```python
from build123d import *

# Parameters (mm, degrees)
SKETCH1_W           = 65
SKETCH1_H           = 16
BOSS_EXTRUDE1_DEPTH = 2
SKETCH2_W           = 65
SKETCH2_H           = 16
SKETCH2_W_2         = 61
SKETCH2_H_2         = 12
BOSS_EXTRUDE2_DEPTH = 2
SKETCH4_W           = 65
SKETCH4_H           = 16
SKETCH4_W_2         = 61
SKETCH4_H_2         = 8
BOSS_EXTRUDE3_DEPTH = 2
SKETCH5_R           = 1
CUT_EXTRUDE1_DEPTH  = 1


with BuildPart() as part:
    # Sketch1 → Boss-Extrude1 (new body)
    with BuildSketch(Plane.XY):
        Rectangle(SKETCH1_W, SKETCH1_H)
    extrude(amount=BOSS_EXTRUDE1_DEPTH)

    # Sketch2 → Boss-Extrude2 (add)
    with BuildSketch(Plane.XY.offset(2)):
        Rectangle(SKETCH2_W, SKETCH2_H)
        Rectangle(SKETCH2_W_2, SKETCH2_H_2, mode=Mode.SUBTRACT)
    extrude(amount=BOSS_EXTRUDE2_DEPTH)

    # Sketch4 → Boss-Extrude3 (add)
    with BuildSketch(Plane.XY.offset(4)):
        Rectangle(SKETCH4_W, SKETCH4_H)
        Rectangle(SKETCH4_W_2, SKETCH4_H_2, mode=Mode.SUBTRACT)
    extrude(amount=BOSS_EXTRUDE3_DEPTH)

    # Sketch5 → Cut-Extrude1 (cut)
    with BuildSketch(Plane.XY.offset(2)):
        with Locations((-26.5, 0)):
            Circle(SKETCH5_R)
    extrude(amount=-CUT_EXTRUDE1_DEPTH, mode=Mode.SUBTRACT)


solid = part.part
```
Design review of the part built by this model. Coordinates are the model's own, in mm. A direction names the side the tool comes from. Round coordinates to 2 decimals unless told otherwise and drop trailing zeros. Write each loop counter-clockwise with the first axis right and the second up, starting at its lowest first coordinate (ties: lowest second). Pieces come first, ordered by that corner, then holes. Notation, with made-up numbers: (-35.75, -38.75) -> (1.25, -38.75) arc R14 cw to (1.25, -31.75) -> close; hole circle Ø3 at (-25, 38.5). An arc over 180 degrees is marked (long way). Answer in a Markdown table with one row per item.
Q1. Clearance check with a flat-ended pin moving along its axis: pin 1 Ø1 at (x, y) = (-26.5, 0) entering from +Z. State where the tip first meets the part, or that it passes through.
The answers:
| item | result |
|---|---|
| pin 1 | z = 1 |
Q2. To check wall thickness, follow L1, parallel to Y at x = 12.5, z = 2.8; L2, parallel to Z at x = -20.5, y = -5; L3, parallel to Y at x = -26.5, z = 1.7. State the ranges of each line that lie inside material, in increasing order. Write a range as [from, to].
The answers:
| item | result |
|---|---|
| L1 | [-8, -6], [6, 8] |
| L2 | [0, 2], [4, 6] |
| L3 | [-8, -1], [1, 8] |
Q3. Take a section at A-A, the plane y = -3. State the section outline as (x, z) points, then the cut area to 3 significant figures.
The answers:
| item | result |
|---|---|
| outline | (-32.5, 0) -> (32.5, 0) -> (32.5, 6) -> (30.5, 6) -> (30.5, 2) -> (-30.5, 2) -> (-30.5, 6) -> (-32.5, 6) -> close |
| area | 146 mm² |
Q4. For faces 1 (the face through (0, 5, 4)), 2 (the face through (-27.5, 0, 1.5)), 3 (the face through (-32.5, 0, 3)), list the 3-axis set-ups (+Z, -Z, +X, -X, +Y, -Y) from which the entire face can be reached by the end or side of a thin tool; tool diameter is ignored.
The answers:
| item | result |
|---|---|
| face 1 | none |
| face 2 | +Z |
| face 3 | +Z, -Z, -X, +Y, -Y |
Q5. Take a section at C-C, the plane x = -26.5. State the section outline as (y, z) points.
The answers:
| item | result |
|---|---|
| outline | (-8, 0) -> (8, 0) -> (8, 6) -> (4, 6) -> (4, 4) -> (6, 4) -> (6, 2) -> (1, 2) -> (1, 1) -> (-1, 1) -> (-1, 2) -> (-6, 2) -> (-6, 4) -> (-4, 4) -> (-4, 6) -> (-8, 6) -> close |
Q6. Take a section at D-D, the plane x = -7. State the section outline as (y, z) points, then the cut area to 3 significant figures.
The answers:
| item | result |
|---|---|
| outline | (-8, 0) -> (8, 0) -> (8, 6) -> (4, 6) -> (4, 4) -> (6, 4) -> (6, 2) -> (-6, 2) -> (-6, 4) -> (-4, 4) -> (-4, 6) -> (-8, 6) -> close |
| area | 56.0 mm² |
Q7. Take a section at B-B, the plane z = 5.15. State the section outline as (x, y) points, then the cut area to 3 significant figures.
The answers:
| item | result |
|---|---|
| outline | (-32.5, -8) -> (32.5, -8) -> (32.5, 8) -> (-32.5, 8) -> close; hole (-30.5, -4) -> (30.5, -4) -> (30.5, 4) -> (-30.5, 4) -> close |
| area | 552 mm² |
Q8. Draft analysis for pull direction Y (two halves, no side actions). For faces 4 (the face through (0, -8, 3)), 5 (the face through (0, 8, 3)), 6 (the face through (0, -4, 5)), 7 (the face through (0, 5, 6)), state which applies: +Y half, -Y half, draft (parallel to the pull), parting line (faces both ways), or undercut.
The answers:
| item | result |
|---|---|
| face 4 | -Y half |
| face 5 | +Y half |
| face 6 | undercut |
| face 7 | draft |
